from build123d import *

# Parameters (mm, degrees)
SKETCH1_R           = 49.55
BOSS_EXTRUDE1_DEPTH = 2.36
SKETCH2_R           = 47.95
BOSS_EXTRUDE2_DEPTH = 2.36
SKETCH3_R           = 3.175
SKETCH3_R_2         = 2.38
CUT_EXTRUDE1_DEPTH  = 5.72


with BuildPart() as part:
    # Sketch1 → Boss-Extrude1 (new body)
    with BuildSketch(Plane(origin=(0, 0, 0), x_dir=(1, 0, 0), z_dir=(0, 1, 0))):
        Circle(SKETCH1_R)
    extrude(amount=BOSS_EXTRUDE1_DEPTH)

    # Sketch2 → Boss-Extrude2 (add)
    with BuildSketch(Plane(origin=(0, 2.36, 0), x_dir=(1, 0, 0), z_dir=(0, 1, 0))):
        Circle(SKETCH2_R)
    extrude(amount=BOSS_EXTRUDE2_DEPTH)

    # Sketch3 → Cut-Extrude1 (cut, through all)
    with BuildSketch(Plane.XZ):
        with Locations((25.4, 0)):
            Circle(SKETCH3_R)
        with Locations((-25.4, 0)):
            Circle(SKETCH3_R)
        with Locations((0, 31.75)):
            Circle(SKETCH3_R)
        with Locations((0, -31.75)):
            Circle(SKETCH3_R)
        with Locations((-18, 18)):
            Circle(SKETCH3_R_2)
    extrude(amount=-CUT_EXTRUDE1_DEPTH, mode=Mode.SUBTRACT)


solid = part.part
Can you work these out from the model? Positions are in its coordinate system, mm. Round coordinates to 2 decimals unless told otherwise and drop trailing zeros. Write each loop counter-clockwise with the first axis right and the second up, starting at its lowest first coordinate (ties: lowest second). Pieces come first, ordered by that corner, then holes. Notation, with made-up numbers: (-20, 69) -> (34, 69) arc R15 cw to (34, 76) -> close; hole circle Ø7 at (-5.75, 12). An arc over 180 degrees is marked (long way). Use one line per item in the form item = value. Start each with the question number.
Q1. Imagine slicing it at A-A (x = 25). Please give me the cut outline in (y, z).
Q2. Imagine slicing it at B-B (z = 31.75). Please give me the cut outline in (x, y) (3 decimals), then the cut area to 3 significant figures.
Q3. Imagine slicing it at C-C (z = 0). Please give me the cut outline in (x, y) (3 decimals).
Q4. If I drill on probe 1 along Z at (x, y) = (0, 1.85) (3 decimals); probe 2 along Z at (x, y) = (0, 3.1) (3 decimals); probe 3 along Z at (x, y) = (-18, 2.3), over which ranges is the centre line in solid material (lowest first)? Write a range as [from, to].
Q5. I'm going to push flat-ended pins straight in: P1, Ø1.5, axis at y = 3, z = 21.5, coming from the +X side; P2, Ø4, axis at x = 0, z = -31.75, coming from the -Y side. Where does each tip first touch, or does it pass through?
Q6. Imagine slicing it at D-D (x = 0). Please give me the cut outline in (y, z) (3 decimals).
Q7. We'd pull the mould along Z, two halves only. Please class faces 1 (the face through (-0.69, 2.33, -34.85)), 2 (the face through (-35.34, 3.52, -32.41)), 3 (the face through (-26, 2.36, -41)): +Z half, -Z half, draft (parallel to the pull), parting line (faces both ways), or undercut.
Worked out:
q1.outline = (0, -42.78) -> (2.36, -42.78) -> (2.36, -40.92) -> (4.72, -40.92) -> (4.72, -3.15) -> (0, -3.15) -> close; (0, 3.15) -> (4.72, 3.15) -> (4.72, 40.92) -> (2.36, 40.92) -> (2.36, 42.78) -> (0, 42.78) -> close
q2.outline = (-38.041, 0) -> (-3.175, 0) -> (-3.175, 4.72) -> (-35.932, 4.72) -> (-35.932, 2.36) -> (-38.041, 2.36) -> close; (3.175, 0) -> (38.041, 0) -> (38.041, 2.36) -> (35.932, 2.36) -> (35.932, 4.72) -> (3.175, 4.72) -> close
q2.area = 319 mm^2
q3.outline = (-49.55, 0) -> (-28.575, 0) -> (-28.575, 4.72) -> (-47.95, 4.72) -> (-47.95, 2.36) -> (-49.55, 2.36) -> close; (-22.225, 0) -> (22.225, 0) -> (22.225, 4.72) -> (-22.225, 4.72) -> close; (28.575, 0) -> (49.55, 0) -> (49.55, 2.36) -> (47.95, 2.36) -> (47.95, 4.72) -> (28.575, 4.72) -> close
q4.probe_1 = [-49.55, -34.925], [-28.575, 28.575], [34.925, 49.55]
q4.probe_2 = [-47.95, -34.925], [-28.575, 28.575], [34.925, 47.95]
q4.probe_3 = [-46.16, 15.62], [20.38, 46.16]
q5.P1 = 44.83
q5.P2 = through
q6.outline = (0, -49.55) -> (2.36, -49.55) -> (2.36, -47.95) -> (4.72, -47.95) -> (4.72, -34.925) -> (0, -34.925) -> close; (0, -28.575) -> (4.72, -28.575) -> (4.72, 28.575) -> (0, 28.575) -> close; (0, 34.925) -> (4.72, 34.925) -> (4.72, 47.95) -> (2.36, 47.95) -> (2.36, 49.55) -> (0, 49.55) -> close
q7.face_1 = undercut
q7.face_2 = parting line
q7.face_3 = draft
